Geometry: final body of the model. Coordinates: model frame, mm. Face numbers are marked on the shaded views. Coordinates: 2 decimals unless noted, no trailing zeros. Order: outer loops, then holes, each group sorted by start corner. A loop starts at its lowest first (then second) coordinate and runs counter-clockwise, first axis right, second up. Notation, with made-up numbers: (59.25, 77) - (97.25, 77) arc R31 ccw to (97.25, 116) - close; hole circle Ø5 at (-37, 43). An arc over 180 degrees is marked (long way). Use a Markdown table: item, result. Add a question column.
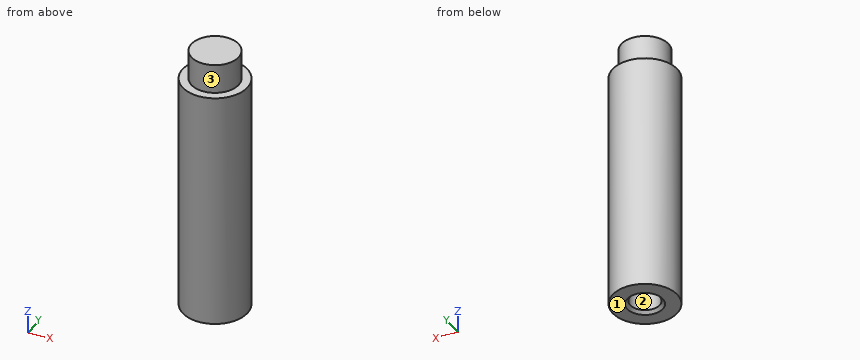
```python
from build123d import *

# Parameters (mm, degrees)
SKETCH1_R                       = 5.5
BOSS_EXTRUDE1_DEPTH             = 40.7
SKETCH2_R                       = 4
BOSS_EXTRUDE2_DEPTH             = 5
M6X1_0_TAPPED_HOLE1_D           = 5
M6X1_0_TAPPED_HOLE1_DEPTH       = 7
M6X1_0_TAPPED_HOLE1_CSINK_D     = 6.05
M6X1_0_TAPPED_HOLE1_CSINK_ANGLE = 90
M6X1_0_TAPPED_HOLE1_TIP         = 1.502151548


with BuildPart() as part:
    # Sketch1 → Boss-Extrude1 (new body)
    with BuildSketch(Plane.XY):
        Circle(SKETCH1_R)
    extrude(amount=BOSS_EXTRUDE1_DEPTH)

    # Sketch2 → Boss-Extrude2 (add)
    with BuildSketch(Plane.XY.offset(40.7)):
        Circle(SKETCH2_R)
    extrude(amount=BOSS_EXTRUDE2_DEPTH)

    # M6x1.0 Tapped Hole1
    with Locations(Plane(origin=(0, 0, 0), x_dir=(-1, 0, 0), z_dir=(0, 0, -1))):
        with Locations((0, 0)):
            CounterSinkHole(M6X1_0_TAPPED_HOLE1_D / 2, M6X1_0_TAPPED_HOLE1_CSINK_D / 2, depth=M6X1_0_TAPPED_HOLE1_DEPTH, counter_sink_angle=M6X1_0_TAPPED_HOLE1_CSINK_ANGLE)
            with Locations((0, 0, -(M6X1_0_TAPPED_HOLE1_DEPTH + M6X1_0_TAPPED_HOLE1_TIP / 2))):  # 118° drill point
                Cone(0, M6X1_0_TAPPED_HOLE1_D / 2, M6X1_0_TAPPED_HOLE1_TIP, mode=Mode.SUBTRACT)


solid = part.part
```
1) First-contact query: pin 1 (1.5 mm diameter, centred on x = 4.5, y = 0, fed in from -Z); pin 2 (1.5 mm diameter, centred on x = 3.5, z = 14.5, fed in from -Y); pin 3 (4 mm diameter, centred on x = 0, y = 0, fed in from -Z). Flat tips, straight axial feed; report the tip coordinate or a pass-through.
2) Draft query along Y for the marked faces 1, 2 and 3. Return one class per face: released by +Y, released by -Y, zero draft, split by the parting line, or undercut.
3) Section query B-B (x = 3.5). Return the cut outline in (y, z), and give its area (3 significant figures).
4) Section query D-D (z = 5). Return the cut outline in (x, y), and give its area (3 significant figures).
5) Section query A-A (z = 33). Return the cut outline in (x, y), and give its area (3 significant figures).
6) Line query: line 1 (Y direction, x = 0, z = 2.75); line 2 (Z direction, x = 3, y = 3.75); line 3 (X direction, y = 0.25, z = 24). Output: solid intervals per line, ascending. Write a range as from..to.
From the geometry:
| question | item | result |
|---|---|---|
| 1 | pin 1 | stops at z = 0 |
| 1 | pin 2 | stops at y = -4.76 |
| 1 | pin 3 | stops at z = 7.3 |
| 2 | face 1 | zero draft |
| 2 | face 2 | undercut |
| 2 | face 3 | split by the parting line |
| 3 | outline | (-4.24, 0) - (4.24, 0) - (4.24, 40.7) - (1.94, 40.7) - (1.94, 45.7) - (-1.94, 45.7) - (-1.94, 40.7) - (-4.24, 40.7) - close |
| 3 | area | 365 mm^2 |
| 4 | outline | circle Ø11 at (0, 0); hole circle Ø5 at (0, 0) |
| 4 | area | 75.4 mm^2 |
| 5 | outline | circle Ø11 at (0, 0) |
| 5 | area | 95.0 mm^2 |
| 6 | line 1 | y = -5.5..-2.5, 2.5..5.5 |
| 6 | line 2 | z = 0..40.7 |
| 6 | line 3 | x = -5.49..5.49 |
